```python
from build123d import *

# Parameters (mm, degrees)
SKETCH_1_R          = 2
SKETCH_1_R_2        = 3
SKETCH_1_R_3        = 2.2
EXTRUDE_1_DEPTH     = 2.5
SKETCH_2_R          = 2
CUT_EXTRUDE_1_DEPTH = 2.5
EXTRUDE_START       = -15
SKETCH_3_R          = 2.2
EXTRUDE_2_DEPTH     = 10


with BuildPart() as part:
    # 草图1 → 凸台-拉伸1 (new, symmetric)
    with BuildSketch(Plane.XY):
        Polygon((0, -20), (60, -20), (100, 0), (100, 20), (60, 40), (0, 40), align=None)
        with Locations((60, 20)):
            Circle(SKETCH_1_R, mode=Mode.SUBTRACT)
        with Locations((60, 0)):
            Circle(SKETCH_1_R, mode=Mode.SUBTRACT)
        with Locations((93, 20)):
            Circle(SKETCH_1_R, mode=Mode.SUBTRACT)
        with Locations((93, 0)):
            Circle(SKETCH_1_R, mode=Mode.SUBTRACT)
        with Locations((45, 0)):
            Circle(SKETCH_1_R_2, mode=Mode.SUBTRACT)
        with Locations((45, 34.2)):
            Circle(SKETCH_1_R_3, mode=Mode.SUBTRACT)
        with Locations((45, -14.2)):
            Circle(SKETCH_1_R_3, mode=Mode.SUBTRACT)
        with Locations((35, 34.2)):
            Circle(SKETCH_1_R_3, mode=Mode.SUBTRACT)
        with Locations((35, -14.2)):
            Circle(SKETCH_1_R_3, mode=Mode.SUBTRACT)
    extrude(amount=EXTRUDE_1_DEPTH, both=True)

    # 草图2 → 切除-拉伸1 (cut, symmetric)
    with BuildSketch(Plane.XY):
        with Locations((80, 10)):
            Circle(SKETCH_2_R)
        with Locations((4, 5)):
            Circle(SKETCH_2_R)
        with Locations((4, 15)):
            Circle(SKETCH_2_R)
    extrude(amount=CUT_EXTRUDE_1_DEPTH, both=True, mode=Mode.SUBTRACT)

    # 草图3 → 凸台-拉伸2 (add)
    # profile 1 of 2: a face of its own
    with BuildSketch(Plane.XY.offset(2.5).offset(EXTRUDE_START)):
        with BuildLine():
            Line((35, 38.2), (45, 38.2))
            ThreePointArc((45, 38.2), (49, 34.2), (45, 30.2))
            Line((45, 30.2), (35, 30.2))
            ThreePointArc((35, 30.2), (31, 34.2), (35, 38.2))
        make_face()
        with Locations((35, 34.2)):
            Circle(SKETCH_3_R, mode=Mode.SUBTRACT)
        with Locations((45, 34.2)):
            Circle(SKETCH_3_R, mode=Mode.SUBTRACT)
    # profile 2 of 2: a face of its own
    with BuildSketch(Plane.XY.offset(2.5).offset(EXTRUDE_START)):
        with BuildLine():
            Line((35, -10.2), (45, -10.2))
            ThreePointArc((45, -10.2), (49, -14.2), (45, -18.2))
            Line((45, -18.2), (35, -18.2))
            ThreePointArc((35, -18.2), (31, -14.2), (35, -10.2))
        make_face()
        with Locations((35, -14.2)):
            Circle(SKETCH_3_R, mode=Mode.SUBTRACT)
        with Locations((45, -14.2)):
            Circle(SKETCH_3_R, mode=Mode.SUBTRACT)
    extrude(amount=EXTRUDE_2_DEPTH)


solid = part.part
```
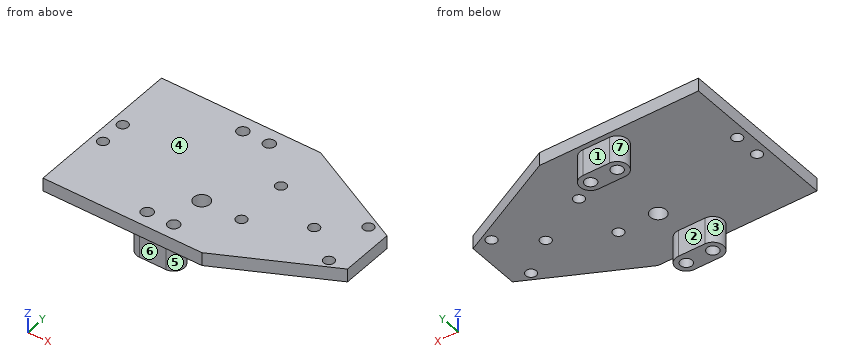
The model under review builds one solid part; all positions refer to its coordinate system, in mm. Face numbers are marked on the shaded views. A direction names the side the tool comes from. Give positions to 0.01 mm unless a question says otherwise; leave off trailing zeros. Write each loop counter-clockwise with the first axis right and the second up, starting at its lowest first coordinate (ties: lowest second). Pieces come first, ordered by that corner, then holes. Notation, with made-up numbers: M -39,1 L -1,1 A13 ccw -1,10 Z; hole C -35.5,49 d7. An arc over 180 degrees is marked long. Write item = value, one per line. Start each with the question number.
Q1. We need section C-C (y = 10). State the section outline as (x, z) points, plus the area to 3 significant figures.
Q2. Machinability: for the marked faces 5, 6 and 7, which of the approach directions +Z, -Z, +X, -X, +Y, -Y give a long, thin tool a straight path to every point of the face, cutting with its end or side? Answer none if there is none.
Q3. We need section D-D (y = -14.2). State the section outline as (x, z) points.
Q4. Mouldability with a two-part tool opening along Y and no side actions: class the marked faces 1, 2, 3 and 4 as released by +Y, released by -Y, zero draft, split by the parting line, or undercut.
Q5. Clearance check with flat-ended pins moving along their axes: pin 1 (3.5 mm diameter, centred on x = 45, y = -14.2, fed in from +Z); pin 2 (8 mm diameter, centred on x = 37, z = -8, fed in from -Y). State where each tip first meets the part, or that it passes through.
Q6. We need section A-A (z = -8.75). State the section outline as (x, y) points.
Q7. For line 1 (Y direction, x = 60, z = 1); line 2 (X direction, y = 34, z = -3.75) (3 decimals); line 3 (Y direction, x = 44.5, z = -6), list the stretches that pass through material, from the lowest coordinate up.
Q8. We need section B-B (x = 93). State the section outline as (y, z) points, plus the area to 3 significant figures.
Result set:
q1.outline = M 0,-2.5 L 78,-2.5 L 78,2.5 L 0,2.5 Z; M 82,-2.5 L 100,-2.5 L 100,2.5 L 82,2.5 Z
q1.area = 480 mm2
q2.face_5 = -Z, +X
q2.face_6 = -Z, +X, -X, -Y
q2.face_7 = -Z, -X
q3.outline = M 0,-2.5 L 31,-2.5 L 31,-12.5 L 32.8,-12.5 L 32.8,2.5 L 0,2.5 Z; M 37.2,-12.5 L 42.8,-12.5 L 42.8,2.5 L 37.2,2.5 Z; M 47.2,-12.5 L 49,-12.5 L 49,-2.5 L 71.6,-2.5 L 71.6,2.5 L 47.2,2.5 Z
q4.face_1 = released by +Y
q4.face_2 = undercut
q4.face_3 = undercut
q4.face_4 = zero draft
q5.pin_1 = through
q5.pin_2 = -18.2
q6.outline = M 35,-18.2 L 45,-18.2 A4 ccw 45,-10.2 L 35,-10.2 A4 ccw Z; M 35,30.2 L 45,30.2 A4 ccw 45,38.2 L 35,38.2 A4 ccw Z; hole C 35,-14.2 d4.4; hole C 35,34.2 d4.4; hole C 45,-14.2 d4.4; hole C 45,34.2 d4.4
q7.line_1 = -20 to -2, 2 to 18, 22 to 40
q7.line_2 = 31.005 to 32.809, 37.191 to 42.809, 47.191 to 48.995
q7.line_3 = -18.2 to -16.34, -12.06 to -10.2, 30.2 to 32.06, 36.34 to 38.2
q8.outline = M -3.5,-2.5 L -2,-2.5 L -2,2.5 L -3.5,2.5 Z; M 2,-2.5 L 18,-2.5 L 18,2.5 L 2,2.5 Z; M 22,-2.5 L 23.5,-2.5 L 23.5,2.5 L 22,2.5 Z
q8.area = 95.0 mm2
